from build123d import *

# Parameters (mm, degrees)
SKETCH1_W                = 20
SKETCH1_H                = 35
BOSS_EXTRUDE1_DEPTH      = 5
SKETCH2_W                = 5.3
SKETCH2_H                = 5
BOSS_EXTRUDE2_DEPTH      = 15
SKETCH3_W                = 10
SKETCH3_H                = 10
CUT_EXTRUDE1_DEPTH       = 1
SKETCH4_W                = 7.35
SKETCH4_H                = 15
CUT_EXTRUDE2_DEPTH       = 21
SKETCH5_W                = 7.35
SKETCH5_H                = 15
CUT_EXTRUDE3_DEPTH       = 21
SKETCH6_W                = 1.5
SKETCH6_H                = 12
BOSS_EXTRUDE3_DEPTH      = 1.85
SKETCH7_W                = 1.5
SKETCH7_H                = 12
BOSS_EXTRUDE4_DEPTH      = 1.85
SKETCH8_W                = 12
SKETCH8_H                = 1.5
BOSS_EXTRUDE5_DEPTH      = 1.85
SKETCH9_W                = 12
SKETCH9_H                = 1.5
BOSS_EXTRUDE6_DEPTH      = 1.85
M3_CLEARANCE_HOLE1_D     = 3.242
M3_CLEARANCE_HOLE1_DEPTH = 20.000025
M3_CLEARANCE_HOLE2_D     = 3.242
M3_CLEARANCE_HOLE2_DEPTH = 5.00005
CHAMFER1_SIZE            = 0.379
FILLET1_R                = 1


with BuildPart() as part:
    # Sketch1 → Boss-Extrude1 (new body)
    with BuildSketch(Plane(origin=(0, 5, 0), x_dir=(1, 0, 0), z_dir=(0, 1, 0))):
        with Locations((0, -17.5)):
            Rectangle(SKETCH1_W, SKETCH1_H)
    extrude(amount=-BOSS_EXTRUDE1_DEPTH)

    # Sketch2 → Boss-Extrude2 (add)
    with BuildSketch(Plane(origin=(0, 5, 0), x_dir=(-1, 0, 0), z_dir=(0, 1, 0))):
        with Locations((0, 2.5)):
            Rectangle(SKETCH2_W, SKETCH2_H)
    extrude(amount=BOSS_EXTRUDE2_DEPTH)

    # Sketch3 → Cut-Extrude1 (cut)
    with BuildSketch(Plane(origin=(0, 5, 0), x_dir=(-1, 0, 0), z_dir=(0, 1, 0))):
        with Locations((0, 10)):
            Rectangle(SKETCH3_W, SKETCH3_H)
    extrude(amount=-CUT_EXTRUDE1_DEPTH, mode=Mode.SUBTRACT)

    # Sketch4 → Cut-Extrude2 (cut, through all)
    with BuildSketch(Plane.XZ):
        with Locations((-6.325, 27.5)):
            Rectangle(SKETCH4_W, SKETCH4_H)
    extrude(amount=-CUT_EXTRUDE2_DEPTH, mode=Mode.SUBTRACT)

    # Sketch5 → Cut-Extrude3 (cut, through all)
    with BuildSketch(Plane.XZ):
        with Locations((6.325, 27.5)):
            Rectangle(SKETCH5_W, SKETCH5_H)
    extrude(amount=-CUT_EXTRUDE3_DEPTH, mode=Mode.SUBTRACT)

    # Sketch6 → Boss-Extrude3 (add)
    with BuildSketch(Plane(origin=(2.65, 0, 0), x_dir=(0, 0, -1), z_dir=(1, 0, 0))):
        with Locations((-2.75, 14)):
            Rectangle(SKETCH6_W, SKETCH6_H)
    extrude(amount=BOSS_EXTRUDE3_DEPTH)

    # Sketch7 → Boss-Extrude4 (add)
    with BuildSketch(Plane.ZY.offset(2.65)):
        with Locations((2.75, 14)):
            Rectangle(SKETCH7_W, SKETCH7_H)
    extrude(amount=BOSS_EXTRUDE4_DEPTH)

    # Sketch8 → Boss-Extrude5 (add)
    with BuildSketch(Plane.ZY.offset(2.65)):
        with Locations((29, 2.75)):
            Rectangle(SKETCH8_W, SKETCH8_H)
    extrude(amount=BOSS_EXTRUDE5_DEPTH)

    # Sketch9 → Boss-Extrude6 (add)
    with BuildSketch(Plane(origin=(2.65, 0, 0), x_dir=(0, 0, -1), z_dir=(1, 0, 0))):
        with Locations((-29, 2.75)):
            Rectangle(SKETCH9_W, SKETCH9_H)
    extrude(amount=BOSS_EXTRUDE6_DEPTH)

    # M3 Clearance Hole1
    with Locations(Plane(origin=(0, 0, 0), x_dir=(-1, 0, 0), z_dir=(0, -1, 0))):
        with Locations((0, -29)):
            Hole(M3_CLEARANCE_HOLE1_D / 2, depth=M3_CLEARANCE_HOLE1_DEPTH)

    # M3 Clearance Hole2
    with Locations(Plane.XY.offset(5)):
        with Locations((0, 14)):
            Hole(M3_CLEARANCE_HOLE2_D / 2, depth=M3_CLEARANCE_HOLE2_DEPTH)

    # Chamfer1
    chamfer1_edges = [part.edges().sort_by_distance(p)[0] for p in [
        (-1.621, 5, 29),
        (-1.621, 0, 29),
        (1.621, 14, 0),
        (1.621, 14, 5),
    ]]
    chamfer(chamfer1_edges, length=CHAMFER1_SIZE)

    # Fillet1
    fillet1_edges = [part.edges().sort_by_distance(p)[0] for p in [
        (-10, 2.5, 20),
        (10, 2.5, 0),
        (10, 2.5, 20),
        (-10, 2.5, 0),
    ]]
    fillet(fillet1_edges, radius=FILLET1_R)


solid = part.part
The model under review builds one solid part; all positions refer to its coordinate system, in mm. A direction names the side the tool comes from. Coordinates: 2 decimals unless noted, no trailing zeros. Write each loop counter-clockwise with the first axis right and the second up, starting at its lowest first coordinate (ties: lowest second). Pieces come first, ordered by that corner, then holes. Notation, with made-up numbers: M 5.25,84.5 L 42.25,84.5 A12 cw 42.25,97.5 Z; hole C -36,57.25 d8. An arc over 180 degrees is marked long. Put each result on its own line as item: value.
1) Add section D-D on z = 3. Give the boundary of the cut face in (x, y), then the cut area to 3 significant figures.
Computed:
outline: M -10,0 L 10,0 L 10,5 L 2.65,5 L 2.65,8 L 4.5,8 L 4.5,20 L -4.5,20 L -4.5,8 L -2.65,8 L -2.65,5 L -10,5 Z; hole C 0,14 d3.24
area: 216 mm2
2) For faces 5 (the flat face through (5, 4.5, 9.9)), 6 (the flat face through (4, 14, 3.5)), 7 (the flat face through (4.5, 14, 3)), 8 (the flat face through (4, 14, 2)), 9 (the flat face through (4, 2, 29)), list the 3-axis set-ups (+Z, -Z, +X, -X, +Y, -Y) from which the entire face can be reached by the end or side of a thin tool; tool diameter is ignored.
Computed:
face 5: +Y
face 6: +Z, +X, +Y
face 7: +Z, -Z, +X, +Y
face 8: -Z, +X, +Y
face 9: +Z, +X, -Y
3) Add section A-A on z = 29. Give the boundary of the cut face in (x, y), then the cut area to 3 significant figures.
Computed:
outline: M -4.5,2 L -2.65,2 L -2.65,0 L -2,0 L -1.62,0.38 L -1.62,4.62 L -2,5 L -2.65,5 L -2.65,3.5 L -4.5,3.5 Z; M 1.62,0.38 L 2,0 L 2.65,0 L 2.65,2 L 4.5,2 L 4.5,3.5 L 2.65,3.5 L 2.65,5 L 2,5 L 1.62,4.62 Z
area: 15.6 mm2
4) Wall thickness on probe 1 along Y at (x, z) = (0, 2.1); probe 2 along Y at (x, z) = (4, 3); probe 3 along Z at (x, y) = (9, 3.75): over which ranges is each line inside the solid? List them lowest first. Write a range as [from, to].
Computed:
probe 1: y = [0, 12.38], [15.62, 20]
probe 2: y = [0, 5], [8, 20]
probe 3: z = [0, 20]
5) Draft analysis for pull direction Z (two halves, no side actions). For faces 1 (the flat face through (4, 3, 23)), 2 (the flat face through (-5, 4.5, 9.9)), 3 (the cylindrical face through (-9.715, 2.465, 0.301)), 4 (the flat face through (10, 3, 10)), state which applies: released by +Z, released by -Z, zero draft, split by the parting line, or undercut.
Computed:
face 1: undercut
face 2: undercut
face 3: released by -Z
face 4: zero draft
6) Add section B-B on x = 0. Give the boundary of the cut face in (y, z), then the cut area to 3 significant figures.
Computed:
outline: M 0,0 L 12,0 L 12.38,0.38 L 12.38,4.62 L 12,5 L 4,5 L 4,15 L 5,15 L 5,27 L 4.62,27.38 L 0.38,27.38 L 0,27 Z; M 0,31 L 0.38,30.62 L 4.62,30.62 L 5,31 L 5,35 L 0,35 Z; M 15.62,0.38 L 16,0 L 20,0 L 20,5 L 16,5 L 15.62,4.62 Z
area: 207 mm2
7) Clearance check with flat-ended pins moving along their axes: pin 1 Ø1.5 at (x, y) = (-6.5, 2.5) entering from +Z; pin 2 Ø8 at (x, y) = (-6, 6) entering from +Z; pin 3 Ø3.5 at (x, y) = (0, 14) entering from +Z; pin 4 Ø6 at (x, y) = (6.5, 14.5) entering from -Z. State where each tip first meets the part, or that it passes through.
Computed:
pin 1: stops at z = 20
pin 2: stops at z = 35
pin 3: stops at z = 4.75
pin 4: stops at z = 2
